Check sheet for the drawn part. Datum: minimum x, y, z corner. Units: mm. A direction names the side the tool comes from. Round coordinates to 2 decimals unless told otherwise and drop trailing zeros. Write each loop counter-clockwise with the first axis right and the second up, starting at its lowest first coordinate (ties: lowest second). Pieces come first, ordered by that corner, then holes. Notation, with made-up numbers: M -10,26.5 L -6,26.5 A21 cw -6,35.5 Z; hole C 4,37.5 d6. An arc over 180 degrees is marked long. Answer in a Markdown table with one row per item. Add a question column.
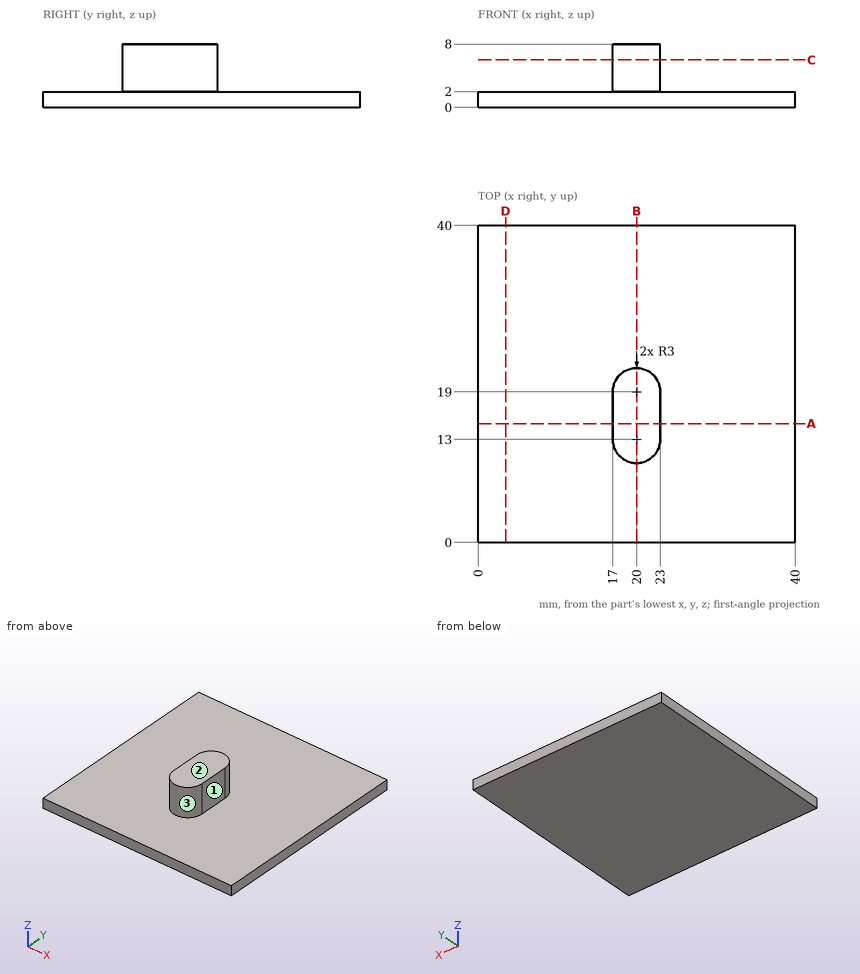
Item 1: Section check D-D, the plane x = 3.5. Record the boundary of the cut face in (y, z), and give its area (3 significant figures).
Item 2: Section check C-C, the plane z = 6. Record the boundary of the cut face in (x, y).
Item 3: Access from +Z, -Z, +X, -X, +Y, -Y to the whole of each face (thin tool, end or side, straight path). Record for the marked faces 1, 2 and 3.
Item 4: Section check A-A, the plane y = 15. Record the boundary of the cut face in (x, z), and give its area (3 significant figures).
Item 5: Gauge pin test, flat ends, axial feed: pin 1 Ø3 at (y, z) = (16.5, 4) entering from +X; pin 2 Ø3 at (x, y) = (4, 22.5) entering from +Z; pin 3 Ø1.5 at (y, z) = (22.5, 5) entering from +X. Record the tip position at first contact, or that the pin passes through.
Item 6: Section check B-B, the plane x = 20. Record the boundary of the cut face in (y, z).
Item 7: Scan lines: probe 1 along Z at (x, y) = (15, 21); probe 2 along X at (y, z) = (16.5, 4.75); probe 3 along Y at (x, z) = (18, 5). Record each from-to range of solid material in increasing order. Write a range as from..to.
Result sheet:
| question | item | result |
|---|---|---|
| 1 | outline | M 0,0 L 40,0 L 40,2 L 0,2 Z |
| 1 | area | 80.0 mm^2 |
| 2 | outline | M 17,13 A3 ccw 23,13 L 23,19 A3 ccw 17,19 Z |
| 3 | face 1 | +Z, +X, +Y, -Y |
| 3 | face 2 | +Z, +X, -X, +Y, -Y |
| 3 | face 3 | +Z, -Y |
| 4 | outline | M 0,0 L 40,0 L 40,2 L 23,2 L 23,8 L 17,8 L 17,2 L 0,2 Z |
| 4 | area | 116 mm^2 |
| 5 | pin 1 | stops at x = 23 |
| 5 | pin 2 | stops at z = 2 |
| 5 | pin 3 | stops at x = 21.2 |
| 6 | outline | M 0,0 L 40,0 L 40,2 L 22,2 L 22,8 L 10,8 L 10,2 L 0,2 Z |
| 7 | probe 1 | z = 0..2 |
| 7 | probe 2 | x = 17..23 |
| 7 | probe 3 | y = 10.76..21.24 |
